```python
from build123d import *

# Parameters (mm, degrees)
SKETCH1_W                           = 17.78
SKETCH1_H                           = 17.78
BOSS_EXTRUDE1_DEPTH                 = 8.89
CHAMFER1_SIZE                       = 0.762
F_7_64_0_10938_DIAMETER_HOLE1_D     = 2.778252
F_7_64_0_10938_DIAMETER_HOLE1_DEPTH = 1.6002
F_7_64_0_10938_DIAMETER_HOLE1_TIP   = 0.834671108
F_7_64_0_10938_DIAMETER_HOLE2_D     = 2.778252
F_7_64_0_10938_DIAMETER_HOLE2_DEPTH = 1.6002
F_7_64_0_10938_DIAMETER_HOLE2_TIP   = 0.834671108
F_7_64_0_10938_DIAMETER_HOLE3_D     = 2.778252
F_7_64_0_10938_DIAMETER_HOLE3_DEPTH = 1.6002
F_7_64_0_10938_DIAMETER_HOLE3_TIP   = 0.834671108
F_7_64_0_10938_DIAMETER_HOLE5_D     = 2.778252
F_7_64_0_10938_DIAMETER_HOLE5_DEPTH = 1.6002
F_7_64_0_10938_DIAMETER_HOLE5_TIP   = 0.834671108
F_7_64_0_10938_DIAMETER_HOLE6_D     = 2.778252
F_7_64_0_10938_DIAMETER_HOLE6_DEPTH = 1.6002
F_7_64_0_10938_DIAMETER_HOLE6_TIP   = 0.834671108
F_7_64_0_10938_DIAMETER_HOLE7_D     = 2.778252
F_7_64_0_10938_DIAMETER_HOLE7_DEPTH = 1.6002
F_7_64_0_10938_DIAMETER_HOLE7_TIP   = 0.834671108


with BuildPart() as part:
    # Sketch1 → Boss-Extrude1 (new, symmetric)
    with BuildSketch(Plane(origin=(0, 0, 0), x_dir=(1, 0, 0), z_dir=(0, 1, 0))):
        Rectangle(SKETCH1_W, SKETCH1_H)
    extrude(amount=BOSS_EXTRUDE1_DEPTH, both=True)

    # Chamfer1
    chamfer1_edges = [part.edges().sort_by_distance(p)[0] for p in [
        (0, 8.89, 8.89),
        (-8.89, 8.89, 0),
        (0, 8.89, -8.89),
        (-8.89, -8.89, 0),
        (0, -8.89, 8.89),
        (8.89, -8.89, 0),
        (0, -8.89, -8.89),
        (8.89, 8.89, 0),
        (-8.89, 0, -8.89),
        (-8.89, 0, 8.89),
        (8.89, 0, 8.89),
        (8.89, 0, -8.89),
    ]]
    chamfer(chamfer1_edges, length=CHAMFER1_SIZE)

    # 7/64 (0.10938) Diameter Hole1
    with Locations(Plane(origin=(0, 8.89, 0), x_dir=(1, 0, 0), z_dir=(0, 1, 0))):
        with Locations((0, 0)):
            Hole(F_7_64_0_10938_DIAMETER_HOLE1_D / 2, depth=F_7_64_0_10938_DIAMETER_HOLE1_DEPTH)
            with Locations((0, 0, -(F_7_64_0_10938_DIAMETER_HOLE1_DEPTH + F_7_64_0_10938_DIAMETER_HOLE1_TIP / 2))):  # 118° drill point
                Cone(0, F_7_64_0_10938_DIAMETER_HOLE1_D / 2, F_7_64_0_10938_DIAMETER_HOLE1_TIP, mode=Mode.SUBTRACT)

    # 7/64 (0.10938) Diameter Hole2
    with Locations(Plane(origin=(0, -8.89, 0), x_dir=(-1, 0, 0), z_dir=(0, -1, 0))):
        with Locations((5.08, -5.08), (5.08, 0), (5.08, 5.08), (-5.08, 5.08), (-5.08, 0), (-5.08, -5.08)):
            Hole(F_7_64_0_10938_DIAMETER_HOLE2_D / 2, depth=F_7_64_0_10938_DIAMETER_HOLE2_DEPTH)
            with Locations((0, 0, -(F_7_64_0_10938_DIAMETER_HOLE2_DEPTH + F_7_64_0_10938_DIAMETER_HOLE2_TIP / 2))):  # 118° drill point
                Cone(0, F_7_64_0_10938_DIAMETER_HOLE2_D / 2, F_7_64_0_10938_DIAMETER_HOLE2_TIP, mode=Mode.SUBTRACT)

    # 7/64 (0.10938) Diameter Hole3
    with Locations(Plane.XY.offset(8.89)):
        with Locations((-5.08, -5.08), (0, 0), (5.08, 5.08)):
            Hole(F_7_64_0_10938_DIAMETER_HOLE3_D / 2, depth=F_7_64_0_10938_DIAMETER_HOLE3_DEPTH)
            with Locations((0, 0, -(F_7_64_0_10938_DIAMETER_HOLE3_DEPTH + F_7_64_0_10938_DIAMETER_HOLE3_TIP / 2))):  # 118° drill point
                Cone(0, F_7_64_0_10938_DIAMETER_HOLE3_D / 2, F_7_64_0_10938_DIAMETER_HOLE3_TIP, mode=Mode.SUBTRACT)

    # 7/64 (0.10938) Diameter Hole5
    with Locations(Plane.ZY.offset(8.89)):
        with Locations((-5.08, 5.08), (5.08, -5.08)):
            Hole(F_7_64_0_10938_DIAMETER_HOLE5_D / 2, depth=F_7_64_0_10938_DIAMETER_HOLE5_DEPTH)
            with Locations((0, 0, -(F_7_64_0_10938_DIAMETER_HOLE5_DEPTH + F_7_64_0_10938_DIAMETER_HOLE5_TIP / 2))):  # 118° drill point
                Cone(0, F_7_64_0_10938_DIAMETER_HOLE5_D / 2, F_7_64_0_10938_DIAMETER_HOLE5_TIP, mode=Mode.SUBTRACT)

    # 7/64 (0.10938) Diameter Hole6
    with Locations(Plane(origin=(8.89, 0, 0), x_dir=(0, 0, -1), z_dir=(1, 0, 0))):
        with Locations((-5.08, 5.08), (-5.08, -5.08), (5.08, -5.08), (5.08, 5.08), (0, 0)):
            Hole(F_7_64_0_10938_DIAMETER_HOLE6_D / 2, depth=F_7_64_0_10938_DIAMETER_HOLE6_DEPTH)
            with Locations((0, 0, -(F_7_64_0_10938_DIAMETER_HOLE6_DEPTH + F_7_64_0_10938_DIAMETER_HOLE6_TIP / 2))):  # 118° drill point
                Cone(0, F_7_64_0_10938_DIAMETER_HOLE6_D / 2, F_7_64_0_10938_DIAMETER_HOLE6_TIP, mode=Mode.SUBTRACT)

    # 7/64 (0.10938) Diameter Hole7
    with Locations(Plane(origin=(0, 0, -8.89), x_dir=(-1, 0, 0), z_dir=(0, 0, -1))):
        with Locations((-5.08, 5.08), (-5.08, -5.08), (5.08, -5.08), (5.08, 5.08)):
            Hole(F_7_64_0_10938_DIAMETER_HOLE7_D / 2, depth=F_7_64_0_10938_DIAMETER_HOLE7_DEPTH)
            with Locations((0, 0, -(F_7_64_0_10938_DIAMETER_HOLE7_DEPTH + F_7_64_0_10938_DIAMETER_HOLE7_TIP / 2))):  # 118° drill point
                Cone(0, F_7_64_0_10938_DIAMETER_HOLE7_D / 2, F_7_64_0_10938_DIAMETER_HOLE7_TIP, mode=Mode.SUBTRACT)


solid = part.part
```
Could you check a few things on this model? Use its own coordinates, in mm. A direction names the side the tool comes from. Coordinates: 2 decimals unless noted, no trailing zeros. Return JSON: item names as keys, results as strings.
(1) Which directions (+Z, -Z, +X, -X, +Y, -Y) give clear straight access to the entire face, cutting with the end or side of a thin tool? Please do faces 1 (the cylindrical face through (6.363, -8.079, 0.532)), 2 (the cylindrical face through (8.079, -3.703, 4.899)), 3 (the cylindrical face through (0.301, 8.079, 1.356)), 4 (the conical face through (5.27, 4.93, -6.6)).
Numbers:
{"face 1": "-Y", "face 2": "+X", "face 3": "+Y", "face 4": "-Z"}
(2) I need wall thicknesses on L1, parallel to Y at x = -5.08, z = -8.05; L2, parallel to X at y = 5.08, z = 7.9; L3, parallel to X at y = -5.08, z = -8.3. Which ranges of each line are inside material? Lowest first, please.
Numbers:
{"L1": "y = -8.89 to -6.47, -3.69 to 3.69, 6.47 to 8.89", "L2": "x = -8.89 to 3.69, 6.47 to 8.89", "L3": "x = -8.72 to -6.47, -3.69 to 3.69, 6.47 to 8.72"}
(3) We'd pull the mould along Y, two halves only. Please class faces 5 (the flat face through (-8.89, 0, 0)), 6 (the flat face through (0, -8.89, 0)), 7 (the conical face through (6.6, 4.93, 5.27)): +Y half, -Y half, draft (parallel to the pull), parting line (faces both ways), or undercut.
Numbers:
{"face 5": "draft", "face 6": "-Y half", "face 7": "undercut"}
(4) I'm going to push flat-ended pins straight in: pin 1 (2 mm diameter, centred on x = 5.08, y = 5.08, fed in from -Z); pin 2 (2.5 mm diameter, centred on y = -5.08, z = 5.08, fed in from +X). Where does each tip first touch, or does it pass through?
Numbers:
{"pin 1": "stops at z = -7.06", "pin 2": "stops at x = 7.21"}
